Can you work these out from the model? Positions are in its coordinate system, mm. Give positions to 0.01 mm unless a question says otherwise; leave off trailing zeros. Loops run counter-clockwise (first coordinate to the right, second up) from the corner with the lowest first, then second, coordinate; pieces in that order, holes last. Notation, with made-up numbers: M 70,-8 L 107,-8 A25 cw 107,11 Z; hole C 82,67.25 d3. An arc over 180 degrees is marked long. Answer as a JSON object with one key per item and string values.
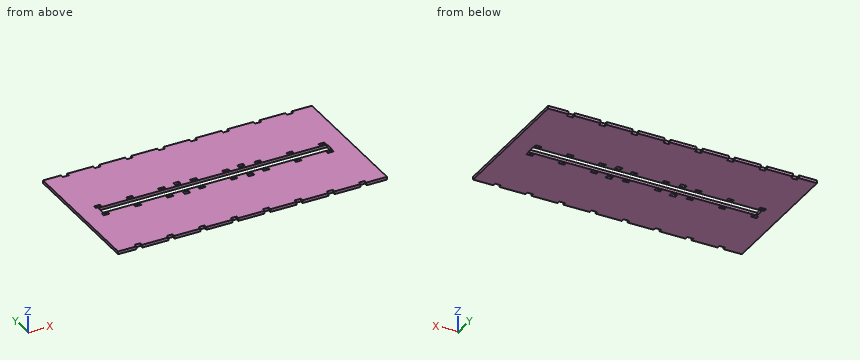
```python
from build123d import *

# Parameters (mm, degrees)
SKETCH4_W                = 298.45
SKETCH4_H                = 38.1
SKETCH4_W_2              = 254
SKETCH4_H_2              = 10.16
BOSS_EXTRUDE1_DEPTH      = 3.175
SKETCH5_W                = 6.604
SKETCH5_H                = 3.429
CUT_EXTRUDE1_DEPTH       = 152.603161408
SKETCH7_W                = 298.45
SKETCH7_H                = 3.175
BOSS_EXTRUDE2_DEPTH      = 57.912
LPATTERN3_COUNT          = 2
LPATTERN3_PITCH          = 67.31
LPATTERN3_COUNT_DIR2     = 8
LPATTERN3_PITCH_DIR2     = 35.56
CUT_EXTRUDE2_DEPTH       = 169.94900264
LPATTERN2_COUNT          = 2
LPATTERN2_PITCH          = 71.12
MIRROR1_COPY_1_SKETCH_W  = 6.604
MIRROR1_COPY_1_SKETCH_H  = 3.429
MIRROR1_COPY_1_DEPTH     = 152.603161408
MIRROR1_COPY_2_SKETCH_W  = 6.604
MIRROR1_COPY_2_SKETCH_H  = 3.429
MIRROR1_COPY_2_DEPTH     = 152.603161408
MIRROR1_COPY_3_SKETCH_W  = 6.604
MIRROR1_COPY_3_SKETCH_H  = 3.429
MIRROR1_COPY_3_DEPTH     = 152.603161408
MIRROR1_COPY_4_SKETCH_W  = 6.604
MIRROR1_COPY_4_SKETCH_H  = 3.429
MIRROR1_COPY_4_DEPTH     = 152.603161408
MIRROR1_COPY_5_SKETCH_W  = 6.604
MIRROR1_COPY_5_SKETCH_H  = 3.429
MIRROR1_COPY_5_DEPTH     = 152.603161408
MIRROR1_COPY_6_SKETCH_W  = 6.604
MIRROR1_COPY_6_SKETCH_H  = 3.429
MIRROR1_COPY_6_DEPTH     = 152.603161408
MIRROR1_COPY_7_SKETCH_W  = 6.604
MIRROR1_COPY_7_SKETCH_H  = 3.429
MIRROR1_COPY_7_DEPTH     = 152.603161408
MIRROR1_COPY_8_SKETCH_W  = 6.604
MIRROR1_COPY_8_SKETCH_H  = 3.429
MIRROR1_COPY_8_DEPTH     = 152.603161408
MIRROR1_COPY_9_SKETCH_W  = 6.604
MIRROR1_COPY_9_SKETCH_H  = 3.429
MIRROR1_COPY_9_DEPTH     = 152.603161408
MIRROR1_COPY_10_SKETCH_W = 6.604
MIRROR1_COPY_10_SKETCH_H = 3.429
MIRROR1_COPY_10_DEPTH    = 152.603161408
MIRROR1_COPY_11_SKETCH_W = 6.604
MIRROR1_COPY_11_SKETCH_H = 3.429
MIRROR1_COPY_11_DEPTH    = 152.603161408
MIRROR1_COPY_12_SKETCH_W = 6.604
MIRROR1_COPY_12_SKETCH_H = 3.429
MIRROR1_COPY_12_DEPTH    = 152.603161408
MIRROR1_COPY_13_SKETCH_W = 6.604
MIRROR1_COPY_13_SKETCH_H = 3.429
MIRROR1_COPY_13_DEPTH    = 152.603161408
MIRROR1_COPY_14_SKETCH_W = 6.604
MIRROR1_COPY_14_SKETCH_H = 3.429
MIRROR1_COPY_14_DEPTH    = 152.603161408
MIRROR1_COPY_15_SKETCH_W = 6.604
MIRROR1_COPY_15_SKETCH_H = 3.429
MIRROR1_COPY_15_DEPTH    = 152.603161408
MIRROR1_COPY_16_DEPTH    = 169.94900264


with BuildPart() as part:
    # Sketch4 → Boss-Extrude1 (new body)
    with BuildSketch(Plane.XY):
        with Locations((-1.143, 0)):
            Rectangle(SKETCH4_W, SKETCH4_H)
        with Locations((-1.143, 0)):
            Rectangle(SKETCH4_W_2, SKETCH4_H_2, mode=Mode.SUBTRACT)
    extrude(amount=BOSS_EXTRUDE1_DEPTH)

    # Sketch5 → Cut-Extrude1 (cut, through all)
    with BuildSketch(Plane.XY.offset(3.175)):
        with Locations((-126.873, 7.9375)):
            Rectangle(SKETCH5_W, SKETCH5_H)
    cut_extrude1 = extrude(amount=-CUT_EXTRUDE1_DEPTH, mode=Mode.SUBTRACT)

    # Sketch7 → Boss-Extrude2 (add)
    with BuildSketch(Plane(origin=(0, 19.05, 0), x_dir=(1, 0, 0), z_dir=(0, 1, 0))):
        with Locations((-1.143, -1.5875)):
            Rectangle(SKETCH7_W, SKETCH7_H)
    boss_extrude2 = extrude(amount=BOSS_EXTRUDE2_DEPTH)

    # LPattern3: Cut-Extrude1 2 × 8
    with Locations(*[(j * LPATTERN3_PITCH_DIR2, i * LPATTERN3_PITCH, 0) for i in range(LPATTERN3_COUNT) for j in range(LPATTERN3_COUNT_DIR2) if (i, j) != (0, 0)]):
        add(cut_extrude1, mode=Mode.SUBTRACT)

    # Sketch6 → Cut-Extrude2 (cut, through all)
    with BuildSketch(Plane(origin=(0, 0, 0), x_dir=(-1, 0, 0), z_dir=(0, 0, -1))):
        Polygon((37.973, 7.9375), (41.148, 7.9375), (41.148, 11.7475), (37.973, 11.7475), (34.798, 11.7475), (34.798, 7.9375), align=None)
    cut_extrude2 = extrude(amount=-CUT_EXTRUDE2_DEPTH, mode=Mode.SUBTRACT)

    # LPattern2: Cut-Extrude2 ×2
    with Locations(*[(i * LPATTERN2_PITCH, 0, 0) for i in range(1, LPATTERN2_COUNT)]):
        add(cut_extrude2, mode=Mode.SUBTRACT)

    # Mirror1: Cut-Extrude1, Boss-Extrude2, Cut-Extrude2 across plane
    add(cut_extrude1.mirror(Plane.ZX), mode=Mode.SUBTRACT)
    add(boss_extrude2.mirror(Plane.ZX))
    add(cut_extrude2.mirror(Plane.ZX), mode=Mode.SUBTRACT)

    # Mirror1 copy 1 sketch → Mirror1 copy 1 (cut, through all)
    with BuildSketch(Plane(origin=(35.56, 0, 3.175), x_dir=(1, 0, 0), z_dir=(0, 0, 1))):
        with Locations((-126.873, -7.9375)):
            Rectangle(MIRROR1_COPY_1_SKETCH_W, MIRROR1_COPY_1_SKETCH_H)
    extrude(amount=-MIRROR1_COPY_1_DEPTH, mode=Mode.SUBTRACT)

    # Mirror1 copy 2 sketch → Mirror1 copy 2 (cut, through all)
    with BuildSketch(Plane(origin=(71.12, 0, 3.175), x_dir=(1, 0, 0), z_dir=(0, 0, 1))):
        with Locations((-126.873, -7.9375)):
            Rectangle(MIRROR1_COPY_2_SKETCH_W, MIRROR1_COPY_2_SKETCH_H)
    extrude(amount=-MIRROR1_COPY_2_DEPTH, mode=Mode.SUBTRACT)

    # Mirror1 copy 3 sketch → Mirror1 copy 3 (cut, through all)
    with BuildSketch(Plane(origin=(106.68, 0, 3.175), x_dir=(1, 0, 0), z_dir=(0, 0, 1))):
        with Locations((-126.873, -7.9375)):
            Rectangle(MIRROR1_COPY_3_SKETCH_W, MIRROR1_COPY_3_SKETCH_H)
    extrude(amount=-MIRROR1_COPY_3_DEPTH, mode=Mode.SUBTRACT)

    # Mirror1 copy 4 sketch → Mirror1 copy 4 (cut, through all)
    with BuildSketch(Plane(origin=(142.24, 0, 3.175), x_dir=(1, 0, 0), z_dir=(0, 0, 1))):
        with Locations((-126.873, -7.9375)):
            Rectangle(MIRROR1_COPY_4_SKETCH_W, MIRROR1_COPY_4_SKETCH_H)
    extrude(amount=-MIRROR1_COPY_4_DEPTH, mode=Mode.SUBTRACT)

    # Mirror1 copy 5 sketch → Mirror1 copy 5 (cut, through all)
    with BuildSketch(Plane(origin=(177.8, 0, 3.175), x_dir=(1, 0, 0), z_dir=(0, 0, 1))):
        with Locations((-126.873, -7.9375)):
            Rectangle(MIRROR1_COPY_5_SKETCH_W, MIRROR1_COPY_5_SKETCH_H)
    extrude(amount=-MIRROR1_COPY_5_DEPTH, mode=Mode.SUBTRACT)

    # Mirror1 copy 6 sketch → Mirror1 copy 6 (cut, through all)
    with BuildSketch(Plane(origin=(213.36, 0, 3.175), x_dir=(1, 0, 0), z_dir=(0, 0, 1))):
        with Locations((-126.873, -7.9375)):
            Rectangle(MIRROR1_COPY_6_SKETCH_W, MIRROR1_COPY_6_SKETCH_H)
    extrude(amount=-MIRROR1_COPY_6_DEPTH, mode=Mode.SUBTRACT)

    # Mirror1 copy 7 sketch → Mirror1 copy 7 (cut, through all)
    with BuildSketch(Plane(origin=(248.92, 0, 3.175), x_dir=(1, 0, 0), z_dir=(0, 0, 1))):
        with Locations((-126.873, -7.9375)):
            Rectangle(MIRROR1_COPY_7_SKETCH_W, MIRROR1_COPY_7_SKETCH_H)
    extrude(amount=-MIRROR1_COPY_7_DEPTH, mode=Mode.SUBTRACT)

    # Mirror1 copy 8 sketch → Mirror1 copy 8 (cut, through all)
    with BuildSketch(Plane(origin=(0, -67.31, 3.175), x_dir=(1, 0, 0), z_dir=(0, 0, 1))):
        with Locations((-126.873, -7.9375)):
            Rectangle(MIRROR1_COPY_8_SKETCH_W, MIRROR1_COPY_8_SKETCH_H)
    extrude(amount=-MIRROR1_COPY_8_DEPTH, mode=Mode.SUBTRACT)

    # Mirror1 copy 9 sketch → Mirror1 copy 9 (cut, through all)
    with BuildSketch(Plane(origin=(35.56, -67.31, 3.175), x_dir=(1, 0, 0), z_dir=(0, 0, 1))):
        with Locations((-126.873, -7.9375)):
            Rectangle(MIRROR1_COPY_9_SKETCH_W, MIRROR1_COPY_9_SKETCH_H)
    extrude(amount=-MIRROR1_COPY_9_DEPTH, mode=Mode.SUBTRACT)

    # Mirror1 copy 10 sketch → Mirror1 copy 10 (cut, through all)
    with BuildSketch(Plane(origin=(71.12, -67.31, 3.175), x_dir=(1, 0, 0), z_dir=(0, 0, 1))):
        with Locations((-126.873, -7.9375)):
            Rectangle(MIRROR1_COPY_10_SKETCH_W, MIRROR1_COPY_10_SKETCH_H)
    extrude(amount=-MIRROR1_COPY_10_DEPTH, mode=Mode.SUBTRACT)

    # Mirror1 copy 11 sketch → Mirror1 copy 11 (cut, through all)
    with BuildSketch(Plane(origin=(106.68, -67.31, 3.175), x_dir=(1, 0, 0), z_dir=(0, 0, 1))):
        with Locations((-126.873, -7.9375)):
            Rectangle(MIRROR1_COPY_11_SKETCH_W, MIRROR1_COPY_11_SKETCH_H)
    extrude(amount=-MIRROR1_COPY_11_DEPTH, mode=Mode.SUBTRACT)

    # Mirror1 copy 12 sketch → Mirror1 copy 12 (cut, through all)
    with BuildSketch(Plane(origin=(142.24, -67.31, 3.175), x_dir=(1, 0, 0), z_dir=(0, 0, 1))):
        with Locations((-126.873, -7.9375)):
            Rectangle(MIRROR1_COPY_12_SKETCH_W, MIRROR1_COPY_12_SKETCH_H)
    extrude(amount=-MIRROR1_COPY_12_DEPTH, mode=Mode.SUBTRACT)

    # Mirror1 copy 13 sketch → Mirror1 copy 13 (cut, through all)
    with BuildSketch(Plane(origin=(177.8, -67.31, 3.175), x_dir=(1, 0, 0), z_dir=(0, 0, 1))):
        with Locations((-126.873, -7.9375)):
            Rectangle(MIRROR1_COPY_13_SKETCH_W, MIRROR1_COPY_13_SKETCH_H)
    extrude(amount=-MIRROR1_COPY_13_DEPTH, mode=Mode.SUBTRACT)

    # Mirror1 copy 14 sketch → Mirror1 copy 14 (cut, through all)
    with BuildSketch(Plane(origin=(213.36, -67.31, 3.175), x_dir=(1, 0, 0), z_dir=(0, 0, 1))):
        with Locations((-126.873, -7.9375)):
            Rectangle(MIRROR1_COPY_14_SKETCH_W, MIRROR1_COPY_14_SKETCH_H)
    extrude(amount=-MIRROR1_COPY_14_DEPTH, mode=Mode.SUBTRACT)

    # Mirror1 copy 15 sketch → Mirror1 copy 15 (cut, through all)
    with BuildSketch(Plane(origin=(248.92, -67.31, 3.175), x_dir=(1, 0, 0), z_dir=(0, 0, 1))):
        with Locations((-126.873, -7.9375)):
            Rectangle(MIRROR1_COPY_15_SKETCH_W, MIRROR1_COPY_15_SKETCH_H)
    extrude(amount=-MIRROR1_COPY_15_DEPTH, mode=Mode.SUBTRACT)

    # Mirror1 copy 16 sketch → Mirror1 copy 16 (cut, through all)
    with BuildSketch(Plane(origin=(71.12, 0, 0), x_dir=(-1, 0, 0), z_dir=(0, 0, -1))):
        Polygon((37.973, -7.9375), (41.148, -7.9375), (41.148, -11.7475), (37.973, -11.7475), (34.798, -11.7475), (34.798, -7.9375), align=None)
    extrude(amount=-MIRROR1_COPY_16_DEPTH, mode=Mode.SUBTRACT)


solid = part.part
```
1) Suppose I cut it at B-B, the plane x = 50.5. Write out the boundary of the cut face in (y, z) (3 decimals), and give its area (3 significant figures).
Answer list:
{"outline": "M -73.533,0 L -9.652,0 L -9.652,3.175 L -73.533,3.175 Z; M -6.223,0 L -5.08,0 L -5.08,3.175 L -6.223,3.175 Z; M 5.08,0 L 6.223,0 L 6.223,3.175 L 5.08,3.175 Z; M 9.652,0 L 73.533,0 L 73.533,3.175 L 9.652,3.175 Z", "area": "413 mm^2"}
2) Please list where these lines run through material, in increasing order: line 1 along Y through (x, z) = (-59, 1.7); line 2 along X through (y, z) = (-10, 1.65); line 3 along X through (y, z) = (2, 1.6). Write a range as from..to.
Answer list:
{"line 1": "-73.53..-9.65, -6.22..-5.08, 5.08..6.22, 9.65..73.53", "line 2": "-150.37..-41.15, -34.8..29.97, 36.32..148.08", "line 3": "-150.37..-128.14, 125.86..148.08"}
3) Suppose I cut it at A-A, the plane x = -12. Write out the boundary of the cut face in (y, z) (3 decimals).
Answer list:
{"outline": "M -76.962,0 L -5.08,0 L -5.08,3.175 L -76.962,3.175 Z; M 5.08,0 L 76.962,0 L 76.962,3.175 L 5.08,3.175 Z"}
4) Will these pins go through, and if not, where does the flat tip stop? pin 1 Ø3 at (x, y) = (-96.5, 57.5) entering from -Z; pin 2 Ø1.6 at (x, z) = (122, 2) entering from +Y.
Answer list:
{"pin 1": "z = 0", "pin 2": "y = 73.53"}
5) Suppose I cut it at C-C, the plane z = 2.65. Give the number of separate pieces and of enclosed holes in the cut face, and give its area (3 significant figures).
Answer list:
{"separate pieces": "1", "enclosed holes": "21", "area": "42,500 mm^2"}
